Geometry check sheet. Reference: the model listing, model coordinates, mm. Round coordinates to 2 decimals unless told otherwise and drop trailing zeros. Order: outer loops, then holes, each group sorted by start corner. A loop starts at its lowest first (then second) coordinate and runs counter-clockwise, first axis right, second up.
(1) Cross-section at A-A on y = 79. Enter the section's corners in (x, z), and give its area (3 significant figures).
(2) Cross-section at B-B on x = 82.5. Enter the section's corners in (y, z).
(3) Cross-section at D-D on z = 7. Count the separate pieces of the cut face and the enclosed holes in it, and give its area (3 significant figures).
(4) Cross-section at C-C on x = 0. Enter the section's corners in (y, z), and give its area (3 significant figures).
(5) Draft check along X on faces 1 (the face through (81, 173, 5)), 2 (the face through (173.986, 167.297, 5.07)), 3 (the face through (1.61, 160.53, 4.93)), 4 (the face through (-9.297, 166.986, 5.07)). Enter one of: pulls with the +X half, pulls with the -X half, needs draft (parallel to the pull), parting line crosses it, or undercut.
(6) Thickness scan on L1, parallel to Y at x = 165, z = 6.75; L2, parallel to X at y = 46.5, z = 4; L3, parallel to X at y = 1, z = 2. Record the ranges inside material, lowest first.
from build123d import *

# Parameters (mm, degrees)
SKETCH1_W           = 195
SKETCH1_H           = 188
SKETCH1_R           = 3
SKETCH1_R_2         = 38
SKETCH1_R_3         = 1.65
BOSS_EXTRUDE1_DEPTH = 10
FILLET1_R           = 20


with BuildPart() as part:
    # Sketch1 → Boss-Extrude1 (new body)
    with BuildSketch(Plane.XY):
        with Locations((82.5, 79)):
            Rectangle(SKETCH1_W, SKETCH1_H)
        with Locations((165, 0)):
            Circle(SKETCH1_R, mode=Mode.SUBTRACT)
        with Locations((165, 158)):
            Circle(SKETCH1_R, mode=Mode.SUBTRACT)
        with Locations((0, 158)):
            Circle(SKETCH1_R, mode=Mode.SUBTRACT)
        Circle(SKETCH1_R, mode=Mode.SUBTRACT)
        with Locations((82.5, 79)):
            Circle(SKETCH1_R_2, mode=Mode.SUBTRACT)
        with Locations((117.168551284, 112.19776426)):
            Circle(SKETCH1_R_3, mode=Mode.SUBTRACT)
        with Locations((47.831448716, 112.19776426)):
            Circle(SKETCH1_R_3, mode=Mode.SUBTRACT)
        with Locations((47.831448716, 45.80223574)):
            Circle(SKETCH1_R_3, mode=Mode.SUBTRACT)
        with Locations((117.168551284, 45.80223574)):
            Circle(SKETCH1_R_3, mode=Mode.SUBTRACT)
    extrude(amount=BOSS_EXTRUDE1_DEPTH)

    # Fillet1
    fillet1_edges = [part.edges().sort_by_distance(p)[0] for p in [
        (-15, 173, 5),
        (180, 173, 5),
        (180, -15, 5),
        (-15, -15, 5),
    ]]
    fillet(fillet1_edges, radius=FILLET1_R)


solid = part.part
Found:
1. outline: (-15, 0) - (44.5, 0) - (44.5, 10) - (-15, 10) - close; (120.5, 0) - (180, 0) - (180, 10) - (120.5, 10) - close
1. area: 1,190 mm2
2. outline: (-15, 0) - (41, 0) - (41, 10) - (-15, 10) - close; (117, 0) - (173, 0) - (173, 10) - (117, 10) - close
3. separate pieces: 1
3. enclosed holes: 9
3. area: 31,600 mm2
4. outline: (-14.36, 0) - (-3, 0) - (-3, 10) - (-14.36, 10) - close; (3, 0) - (155, 0) - (155, 10) - (3, 10) - close; (161, 0) - (172.36, 0) - (172.36, 10) - (161, 10) - close
4. area: 1,750 mm2
5. face 1: needs draft
5. face 2: pulls with the +X half
5. face 3: undercut
5. face 4: pulls with the -X half
6. L1: y = -14.36 to -3, 3 to 155, 161 to 172.36
6. L2: x = -15 to 46.34, 49.33 to 62.81, 102.19 to 115.67, 118.66 to 180
6. L3: x = -14.6 to -2.83, 2.83 to 162.17, 167.83 to 179.6
